Input: part model. Units: mm. Frame: model coordinates. A direction names the side the tool comes from. Coordinates: 2 decimals unless noted, no trailing zeros. Order: outer loops, then holes, each group sorted by start corner. A loop starts at its lowest first (then second) coordinate and runs counter-clockwise, first axis right, second up. Notation, with made-up numbers: (68, 87) -> (81, 87) arc R22 cw to (81, 119) -> close; hole circle Ø9 at (42, 15.5). An arc over 180 degrees is marked (long way). One line per item, written item: value. Start each with the question number.
from build123d import *

# Parameters (mm, degrees)
ESQUISSE1_R        = 8.76
BOSS_EXTRU_1_DEPTH = 22.9
COQUE1_T           = -0.77
CONG_1_R           = 0.25
CONG_2_R           = 0.25
CONG_3_R           = 0.1


with BuildPart() as part:
    # Esquisse1 → Boss.-Extru.1 (new body)
    with BuildSketch(Plane.XY):
        with Locations((-3.305589664, 2.980219473)):
            Circle(ESQUISSE1_R)
    extrude(amount=BOSS_EXTRU_1_DEPTH)

    # Coque1
    coque1_openings = [part.faces().sort_by_distance(p)[0] for p in [
        (-3.305589664, 2.980219473, 22.9),
    ]]
    offset(amount=COQUE1_T, openings=coque1_openings, kind=Kind.INTERSECTION)

    # Congé1
    cong_1_edges = [part.edges().sort_by_distance(p)[0] for p in [
        (-11.295589664, 2.980219473, 0.77),
    ]]
    fillet(cong_1_edges, radius=CONG_1_R)

    # Congé2
    cong_2_edges = [part.edges().sort_by_distance(p)[0] for p in [
        (-12.065589664, 2.980219473, 0),
    ]]
    fillet(cong_2_edges, radius=CONG_2_R)

    # Congé3
    cong_3_edges = [part.edges().sort_by_distance(p)[0] for p in [
        (-12.065589664, 2.980219473, 22.9),
        (-11.295589664, 2.980219473, 22.9),
    ]]
    fillet(cong_3_edges, radius=CONG_3_R)


solid = part.part
1) Ray query, line 1 along Y through (x, z) = (-3, 17.5); line 2 along Z through (x, y) = (-6.75, -3.25); line 3 along X through (y, z) = (2.25, 14). Return the intervals inside material, ascending. Write a range as from..to.
2) Section query A-A, the plane z = 13.25. Return the cut outline in (x, y).
3) Pin query (flat end, axial travel): pin 1 Ø3 at (x, y) = (0.5, 3.5) entering from +Z; pin 2 Ø2 at (x, z) = (-4.5, 15) entering from +Y; pin 3 Ø4 at (y, z) = (8.5, 5.5) entering from +X. Return the tip coordinate at first contact, or that it passes through.
4) Mould query, pull axis X, two halves, no side actions, for faces 1 (the cylindrical face through (0.74, -4.79, 11.37)), 2 (the flat face through (-3, 3, 0.77)), 3 (the flat face through (-11, 6, 22.9)). Classes: +X half, -X half, draft (parallel to the pull), parting line (faces both ways), or undercut.
5) Access query for faces 4 (the cylindrical face through (-9.195, 8.38, 11.758)), 5 (the flat face through (-3, 3, 0)). Directions: +Z, -Z, +X, -X, +Y, -Y. A direction counts if a zero-diameter tool reaches every point of the face in a straight line with its end or side. Return the directions, or none.
Entries:
1. line 1: y = -5.77..-5, 10.96..11.73
1. line 2: z = 0..0.77
1. line 3: x = -12.04..-11.26, 4.65..5.42
2. outline: circle Ø17.52 at (-3.31, 2.98); hole circle Ø15.98 at (-3.31, 2.98)
3. pin 1: stops at z = 0.77
3. pin 2: stops at y = 11.74
3. pin 3: stops at x = 4.72
4. face 1: parting line
4. face 2: undercut
4. face 3: draft
5. face 4: +Z
5. face 5: -Z, +X, -X, +Y, -Y
